Verification items for the finished model (mm, model axes). A direction names the side the tool comes from. Round coordinates to 2 decimals unless told otherwise and drop trailing zeros. Write each loop counter-clockwise with the first axis right and the second up, starting at its lowest first coordinate (ties: lowest second). Pieces come first, ordered by that corner, then holes. Notation, with made-up numbers: (41, 57) - (49, 57) arc R23 ccw to (49, 82) - close; hole circle Ø8 at (-3, -15.75). An arc over 180 degrees is marked (long way). Answer as a JSON object with one key per item and string values.
```python
from build123d import *

# Parameters (mm, degrees)
BOSS_EXTRUDE1_DEPTH   = 3.175
F_2_CLEARANCE_HOLE1_D = 2.2606
SKETCH4_W             = 3.175
SKETCH4_H             = 19.05
SKETCH4_W_2           = 19.05
SKETCH4_H_2           = 3.175
CUT_EXTRUDE1_DEPTH    = 72.01498393


with BuildPart() as part:
    # Sketch1 → Boss-Extrude1 (new body)
    with BuildSketch(Plane(origin=(0, 0, 0), x_dir=(1, 0, 0), z_dir=(0, 1, 0))):
        Polygon((-19.463895296, 46.99), (-9.525027315, 46.99), (-9.525027315, 50.165), (9.524972685, 50.165), (9.524972685, 46.990031352), (19.463840666, 46.990031352), (26.491681613, 39.962190405), (28.736745643, 42.207254435), (42.207129825, 28.736870254), (39.962087963, 26.491828392), (46.98992891, 19.463987446), (46.98992891, 9.525119465), (50.16492891, 9.525119465), (50.16492891, -9.524880535), (46.989960262, -9.524880535), (46.989960262, -19.463748516), (39.962119315, -26.491589463), (42.207183345, -28.736653493), (28.736799164, -42.207037675), (26.491757302, -39.961995814), (19.463916356, -46.98983676), (9.525048375, -46.98983676), (9.525048375, -50.16483676), (-9.524951625, -50.16483676), (-9.524951625, -46.989868112), (-19.463819606, -46.989868112), (-26.491660553, -39.962027165), (-28.736724583, -42.207091196), (-42.207108765, -28.736707014), (-39.962066904, -26.491665153), (-46.98990785, -19.463824206), (-46.98990785, -9.524956225), (-50.16490785, -9.524956225), (-50.16490785, 9.525043775), (-46.989939202, 9.525043775), (-46.989939202, 19.463911756), (-39.962098255, 26.491752703), (-42.207162286, 28.736816733), (-28.736778104, 42.207200915), (-26.491736243, 39.962159053), align=None)
    extrude(amount=BOSS_EXTRUDE1_DEPTH)

    # #2 Clearance Hole1 (through all)
    with Locations(Plane(origin=(0, 3.175, 0), x_dir=(1, 0, 0), z_dir=(0, 1, 0))):
        with Locations((-29.718, -26.781346139), (-29.718, 32.541008543), (29.718, 32.541008543), (29.718, -26.781346139)):
            Hole(F_2_CLEARANCE_HOLE1_D / 2)

    # Sketch4 → Cut-Extrude1 (cut, through all)
    with BuildSketch(Plane(origin=(0, 3.175, 0), x_dir=(1, 0, 0), z_dir=(0, 1, 0))):
        with Locations((-24.4475, -0.746346139)):
            Rectangle(SKETCH4_W, SKETCH4_H)
        with Locations((24.4475, -0.746346139)):
            Rectangle(SKETCH4_W, SKETCH4_H)
        with Locations((0, 18.938653861)):
            Rectangle(SKETCH4_W_2, SKETCH4_H_2)
        with Locations((0, -25.193846139)):
            Rectangle(SKETCH4_W_2, SKETCH4_H_2)
    extrude(amount=-CUT_EXTRUDE1_DEPTH, mode=Mode.SUBTRACT)


solid = part.part
```
1. Access from +Z, -Z, +X, -X, +Y, -Y to the whole of each face (thin tool, end or side, straight path). Record for faces 1 (the face through (-27.63, 1.57, -41.1)), 2 (the face through (26.035, 2, 1)), 3 (the face through (41.1, 1.57, -27.63)), 4 (the face through (-14, 2, 46.99)), 5 (the face through (9.525, 2, 49)).
Completed:
{"face 1": "-Z, +Y, -Y", "face 2": "+Y, -Y", "face 3": "+X, +Y, -Y", "face 4": "+Z, -X, +Y, -Y", "face 5": "+Z, +X, +Y, -Y"}
2. Go/stop test with flat-tipped pins: pin 1 (1 mm diameter, centred on x = 48, y = 2, fed in from +Z); pin 2 (3 mm diameter, centred on x = 29.72, z = 26.78, fed in from -Y); pin 3 (1.6 mm diameter, centred on x = 48.5, y = 2, fed in from -Z); pin 4 (1 mm diameter, centred on y = 2, z = 12, fed in from +X). Record where each tip stops, or that it passes through.
Completed:
{"pin 1": "stops at z = 9.52", "pin 2": "stops at y = 0", "pin 3": "stops at z = -9.53", "pin 4": "stops at x = 46.99"}
3. Cross-section at B-B (x = 5). Record the boundary of the cut face in (y, z) (3 decimals).
Completed:
{"outline": "(0, -50.165) - (3.175, -50.165) - (3.175, -20.526) - (0, -20.526) - close; (0, -17.351) - (3.175, -17.351) - (3.175, 23.606) - (0, 23.606) - close; (0, 26.781) - (3.175, 26.781) - (3.175, 50.165) - (0, 50.165) - close"}
4. Material ranges on probe 1 along Z at (x, y) = (6, 2) (3 decimals); probe 2 along X at (y, z) = (0.6, -8) (3 decimals); probe 3 along X at (y, z) = (0.85, -33), recorded low to high. Write a range as from..to.
Completed:
{"probe 1": "z = -50.165..-20.526, -17.351..23.606, 26.781..50.165", "probe 2": "x = -50.165..-26.035, -22.86..22.86, 26.035..50.165", "probe 3": "x = -37.94..-30.75, -28.69..28.69, 30.75..37.94"}
5. Mould release check, pull along Z, two halves, no side actions. Record for faces 6 (the face through (1, 0, -1)), 7 (the face through (-9.525, 2, -19)), 8 (the face through (-22.929, 1.565, 43.525)): released by +Z, released by -Z, zero draft, split by the parting line, or undercut.
Completed:
{"face 6": "zero draft", "face 7": "undercut", "face 8": "released by +Z"}
6. Cross-section at A-A (z = 6). Record the boundary of the cut face in (x, y) (3 decimals).
Completed:
{"outline": "(-50.165, 0) - (-26.035, 0) - (-26.035, 3.175) - (-50.165, 3.175) - close; (-22.86, 0) - (22.86, 0) - (22.86, 3.175) - (-22.86, 3.175) - close; (26.035, 0) - (50.165, 0) - (50.165, 3.175) - (26.035, 3.175) - close"}
7. Cross-section at C-C (x = -17). Record the boundary of the cut face in (y, z) (3 decimals).
Completed:
{"outline": "(0, -46.99) - (3.175, -46.99) - (3.175, 46.99) - (0, 46.99) - close"}
8. Cross-section at D-D (y = 0.7). Count the separate pieces of the cut face and the enclosed holes in it, plus the area to 3 significant figures.
Completed:
{"separate pieces": "1", "enclosed holes": "8", "area": "7,540 mm^2"}
